Source: CAD feature listing. Evaluate the final solid. Frame: model axes, mm. A direction names the side the tool comes from. Give positions to 0.01 mm unless a question says otherwise; leave off trailing zeros. Order: outer loops, then holes, each group sorted by start corner. A loop starts at its lowest first (then second) coordinate and runs counter-clockwise, first axis right, second up. Notation, with made-up numbers: M -2.75,37.5 L 32.25,37.5 A27 ccw 32.25,67.5 Z; hole C -28.75,88 d7. An arc over 180 degrees is marked long. Answer as a JSON object with one key per item and string values. Group by question number.
1. Section query A-A (x = 0). Output: boundary loops of the cut face in (y, z), plus the area to 3 significant figures.
2. Section query C-C (z = 6). Output: boundary loops of the cut face in (x, y), plus the area to 3 significant figures.
3. Section query B-B (z = -1). Output: boundary loops of the cut face in (x, y).
4. Pin query (flat end, axial travel): P1, Ø1, axis at x = -22.5, y = 3.5, coming from the -Z side; P2, Ø3.5, axis at x = 6, z = 0, coming from the -Y side; P3, Ø5, axis at x = 0, z = -6, coming from the +Y side; P4, Ø1, axis at x = -10, y = 0.5, coming from the +Z side. Return the tip coordinate at first contact, or that it passes through.
5. Section query D-D (y = 1.75). Output: boundary loops of the cut face in (x, z).
6. Material intervals for L1, parallel to Z at x = 0, y = 1.4; L2, parallel to Y at x = 23, z = -22; L3, parallel to Z at x = 0, y = 5.8, sorted ascending. Write a range as [from, to].
7. Pull-direction query (Z, two-part tool) for faces 4 (the cylindrical face through (-0.09, 2.46, -8.15)), 5 (the cylindrical face through (-31, 0.49, -9.76)), 6 (the flat face through (-9, 1, -29)); classes: +Z half, -Z half, draft (parallel to the pull), parting line (faces both ways), or undercut.
8. Set-up query: faces 1 (the cylindrical face through (-1.269, 5.76, -9.667)), 2 (the cylindrical face through (-29.97, 3.22, 1.32)), 3 (the cylindrical face through (-0.09, 2.46, 3.85)). Return all of +Z, -Z, +X, -X, +Y, -Y with unobstructed straight access to the full face (end or side cutting, diameter ignored); none if empty.
Autodesk Inventor part; units mm, degrees
ref_plane "YZ Plane" through (0, 0, 0) normal (1, 0, 0) x (0, 1, 0)
ref_plane "XZ Plane" through (0, 0, 0) normal (0, 1, 0) x (-1, 0, 0)
ref_plane "XY Plane" through (0, 0, 0) normal (0, 0, 1) x (1, 0, 0)
sketch "Sketch1" plane through (0, 0, 0) normal (0, 1, 0) x (-1, 0, 0)
  circle A0 centre (0, 0) radius 32.5
  dimension "d0" = 65
extrude "Extrusion1" add sketch "Sketch1" along normal blind 1
sketch "Sketch2" plane through (0, 1, 0) normal (0, 1, 0) x (1, 0, 0)
  circle A0 centre (0, 0) radius 30
  dimension "d3" = 60
extrude "Extrusion2" add sketch "Sketch2" along normal blind 4.5
sketch "Sketch3" plane through (0, 5.5, 0) normal (0, 1, 0) x (1, 0, 0)
  circle A0 centre (0, 0) radius 32.5
  dimension "d6" = 65
extrude "Extrusion3" add sketch "Sketch3" along normal blind 1
sketch "Sketch4" plane through (0, 6.5, 0) normal (0, 1, 0) x (1, 0, 0)
  circle A0 centre (0, 0) radius 9.75
  dimension "d9" = 19.5
extrude "Extrusion4" cut sketch "Sketch4" against normal blind 1.5
sketch "Sketch5" plane through (0, 5, 0) normal (0, 1, 0) x (1, 0, 0)
  circle A0 centre (0, 6) radius 2.15
  circle A1 centre (0, -6) radius 2.15
  circle A2 centre (-6, 0) radius 2.15
  circle A3 centre (6, 0) radius 2.15
  point P0 (0, 0)
  dimension "d12" = 4.3
  dimension "d13" = 6
  dimension "d14" = 4.3
  dimension "d15" = 12
  dimension "d16" = 4.3
  dimension "d17" = 6
  dimension "d18" = 4.3
  dimension "d19" = 12
hole "Hole1" at (0, 5, -6) at (6, 5, 0) at (0, 5, 6) at (-6, 5, 0) direction (0, -1, 0) diameter 4.3 end through all
properties part number "LargeWheel"
Answer sheet:
{
 "1": {"outline": "M 0,-32.5 L 1,-32.5 L 1,-30 L 5.5,-30 L 5.5,-32.5 L 6.5,-32.5 L 6.5,-9.75 L 5,-9.75 L 5,-8.15 L 0,-8.15 Z; M 0,-3.85 L 5,-3.85 L 5,3.85 L 0,3.85 Z; M 0,8.15 L 5,8.15 L 5,9.75 L 6.5,9.75 L 6.5,32.5 L 5.5,32.5 L 5.5,30 L 1,30 L 1,32.5 L 0,32.5 Z", "area": "328 mm^2"},
 "2": {"outline": "M -31.94,0 L -2.15,0 L -2.15,5 L -7.69,5 L -7.69,6.5 L -31.94,6.5 L -31.94,5.5 L -29.39,5.5 L -29.39,1 L -31.94,1 Z; M 2.15,0 L 31.94,0 L 31.94,1 L 29.39,1 L 29.39,5.5 L 31.94,5.5 L 31.94,6.5 L 7.69,6.5 L 7.69,5 L 2.15,5 Z", "area": "348 mm^2"},
 "3": {"outline": "M -32.48,0 L -7.9,0 L -7.9,5 L -9.7,5 L -9.7,6.5 L -32.48,6.5 L -32.48,5.5 L -29.98,5.5 L -29.98,1 L -32.48,1 Z; M -4.1,0 L 4.1,0 L 4.1,5 L -4.1,5 Z; M 7.9,0 L 32.48,0 L 32.48,1 L 29.98,1 L 29.98,5.5 L 32.48,5.5 L 32.48,6.5 L 9.7,6.5 L 9.7,5 L 7.9,5 Z"},
 "4": {"P1": "z = -20.4", "P2": "through", "P3": "y = 5", "P4": "z = 31.08"},
 "5": {"outline": "C 0,0 d60; hole C -6,0 d4.3; hole C 0,-6 d4.3; hole C 0,6 d4.3; hole C 6,0 d4.3"},
 "6": {"L1": "[-30, -8.15], [-3.85, 3.85], [8.15, 30]", "L2": "[0, 1], [5.5, 6.5]", "L3": "[-32.5, -9.75], [9.75, 32.5]"},
 "7": {"face 4": "undercut", "face 5": "parting line", "face 6": "draft"},
 "8": {"face 1": "+Y", "face 2": "none", "face 3": "+Y, -Y"}
}
